from build123d import *

# Parameters (mm, degrees)
SKETCH1_W           = 33.8
SKETCH1_H           = 18
BOSS_EXTRUDE1_DEPTH = 7
SKETCH2_W           = 1.5
SKETCH2_H           = 18
BOSS_EXTRUDE2_DEPTH = 15
SKETCH3_R           = 1.4
CUT_EXTRUDE1_DEPTH  = 34.8
FILLET1_R           = 6


with BuildPart() as part:
    # Sketch1 → Boss-Extrude1 (new body)
    with BuildSketch(Plane.XY):
        Rectangle(SKETCH1_W, SKETCH1_H)
        with BuildLine():
            Line((-5, 3.5), (-5, -3.5))
            ThreePointArc((-5, -3.5), (-9, -7.5), (-13, -3.5))
            Line((-13, -3.5), (-13, 3.5))
            ThreePointArc((-13, 3.5), (-9, 7.5), (-5, 3.5))
        make_face(mode=Mode.SUBTRACT)
        with BuildLine():
            Line((13, 3.5), (13, -3.5))
            ThreePointArc((13, -3.5), (9, -7.5), (5, -3.5))
            Line((5, -3.5), (5, 3.5))
            ThreePointArc((5, 3.5), (9, 7.5), (13, 3.5))
        make_face(mode=Mode.SUBTRACT)
    extrude(amount=BOSS_EXTRUDE1_DEPTH)

    # Sketch2 → Boss-Extrude2 (add)
    with BuildSketch(Plane.XY.offset(7)):
        with Locations((-16.15, 0)):
            Rectangle(SKETCH2_W, SKETCH2_H)
        with Locations((16.15, 0)):
            Rectangle(SKETCH2_W, SKETCH2_H)
    extrude(amount=BOSS_EXTRUDE2_DEPTH)

    # Sketch3 → Cut-Extrude1 (cut, through all)
    with BuildSketch(Plane(origin=(16.9, 0, 0), x_dir=(0, 0, -1), z_dir=(1, 0, 0))):
        with Locations((-19.1, 0)):
            Circle(SKETCH3_R)
    extrude(amount=-CUT_EXTRUDE1_DEPTH, mode=Mode.SUBTRACT)

    # Fillet1
    fillet1_edges = [part.edges().sort_by_distance(p)[0] for p in [
        (16.15, -9, 22),
        (-16.15, -9, 22),
        (-16.15, 9, 22),
        (16.15, 9, 22),
    ]]
    fillet(fillet1_edges, radius=FILLET1_R)


solid = part.part
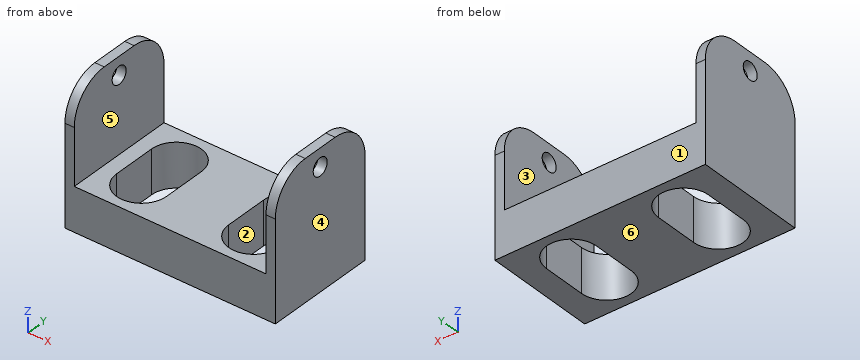
Design review of the part built by this model. Coordinates are the model's own, in mm. Face numbers are marked on the shaded views. A direction names the side the tool comes from. Coordinates: 2 decimals unless noted, no trailing zeros. Order: outer loops, then holes, each group sorted by start corner. A loop starts at its lowest first (then second) coordinate and runs counter-clockwise, first axis right, second up. Notation, with made-up numbers: (39.5, 71.5) -> (48.5, 71.5) arc R25 ccw to (48.5, 91.5) -> close; hole circle Ø11 at (44, 37). An arc over 180 degrees is marked (long way). Use one line per item in the form item = value. Start each with the question number.
(1) Add section D-D on x = 9. State the section outline as (y, z) points, plus the area to 3 significant figures.
(2) The part is to be moulded in two halves that separate along X. For the marked faces 4, 5 and 6, say which applies: +X half, -X half, draft (parallel to the pull), parting line (faces both ways), or undercut.
(3) Add section C-C on y = 0. State the section outline as (x, z) points, plus the area to 3 significant figures.
(4) Add section A-A on y = 2.25. State the section outline as (x, z) points.
(5) For probe 1 along X at (y, z) = (0.25, 3); probe 2 along X at (y, z) = (-3.75, 14.75); probe 3 along X at (y, z) = (-5.25, 2.25), list the stretches that pass through material, from the lowest coordinate up.
(6) Insertion check: pin 1 (4 mm diameter, centred on x = 11.5, y = 0, fed in from +Z). The pin has a flat end and moves straight along its axis. Give the tip position at first contact, or say it passes through.
(7) Add section B-B on z = 11. State the section outline as (x, y) points.
(8) For the marked faces 1, 2 and 3, list the 3-axis set-ups (+Z, -Z, +X, -X, +Y, -Y) from which the entire face can be reached by the end or side of a thin tool; tool diameter is ignored.
Answer block:
q1.outline = (-9, 0) -> (-7.5, 0) -> (-7.5, 7) -> (-9, 7) -> close; (7.5, 0) -> (9, 0) -> (9, 7) -> (7.5, 7) -> close
q1.area = 21.0 mm²
q2.face_4 = +X half
q2.face_5 = undercut
q2.face_6 = draft
q3.outline = (-16.9, 0) -> (-13, 0) -> (-13, 7) -> (-15.4, 7) -> (-15.4, 17.7) -> (-16.9, 17.7) -> close; (-16.9, 20.5) -> (-15.4, 20.5) -> (-15.4, 22) -> (-16.9, 22) -> close; (-5, 0) -> (5, 0) -> (5, 7) -> (-5, 7) -> close; (13, 0) -> (16.9, 0) -> (16.9, 17.7) -> (15.4, 17.7) -> (15.4, 7) -> (13, 7) -> close; (15.4, 20.5) -> (16.9, 20.5) -> (16.9, 22) -> (15.4, 22) -> close
q3.area = 161 mm²
q4.outline = (-16.9, 0) -> (-13, 0) -> (-13, 7) -> (-15.4, 7) -> (-15.4, 22) -> (-16.9, 22) -> close; (-5, 0) -> (5, 0) -> (5, 7) -> (-5, 7) -> close; (13, 0) -> (16.9, 0) -> (16.9, 22) -> (15.4, 22) -> (15.4, 7) -> (13, 7) -> close
q5.probe_1 = -16.9 to -13, -5 to 5, 13 to 16.9
q5.probe_2 = -16.9 to -15.4, 15.4 to 16.9
q5.probe_3 = -16.9 to -12.6, -5.4 to 5.4, 12.6 to 16.9
q6.pin_1 = 7
q7.outline = (-16.9, -9) -> (-15.4, -9) -> (-15.4, 9) -> (-16.9, 9) -> close; (15.4, -9) -> (16.9, -9) -> (16.9, 9) -> (15.4, 9) -> close
q8.face_1 = +Z, -Z, +X, -X, +Y
q8.face_2 = +Z, -Z
q8.face_3 = +Z, +Y, -Y
